from build123d import *

# Parameters (mm, degrees)
BOSS_EXTRUDE1_DEPTH = 0.5
BOSS_EXTRUDE6_DEPTH = 5
BOSS_EXTRUDE5_DEPTH = 6.75
LPATTERN2_COUNT     = 2
LPATTERN2_PITCH     = 13.75
CUT_EXTRUDE4_REACH  = 84.156
SKETCH10_R          = 1.75
LPATTERN3_COUNT     = 2
LPATTERN3_PITCH     = 12
CUT_EXTRUDE5_REACH  = 84.156
SKETCH12_R          = 1.25
SKETCH13_W          = 7
SKETCH13_H          = 6
CUT_EXTRUDE6_DEPTH  = 1
CHAMFER1_SIZE       = 5
CUT_EXTRUDE8_REACH  = 84.105
SKETCH15_W          = 10
SKETCH15_H          = 3
CUT_EXTRUDE9_REACH  = 84.032
SKETCH16_W          = 3
SKETCH16_H          = 7


with BuildPart() as part:
    # Sketch1 → Boss-Extrude1 (new, symmetric)
    with BuildSketch(Plane.XY):
        with BuildLine():
            Line((-56.5, -6), (27.587658385, -6))
            Line((27.587658385, -6), (27.587658385, 0))
            ThreePointArc((27.587658385, 0), (37.034297035, 20.970760182), (59, 27.791292246))
            Line((59, 27.791292246), (76, 25.703954711))
            Line((76, 25.703954711), (76, 30.62))
            Line((76, 30.62), (0, 30.62))
            Line((0, 30.62), (0, -2.5))
            Line((0, -2.5), (-56.5, -2.5))
            Line((-56.5, -2.5), (-56.5, -6))
        make_face()
    extrude(amount=BOSS_EXTRUDE1_DEPTH, both=True)

    # Sketch5 → Boss-Extrude6 (add)
    with BuildSketch(Plane(origin=(0, 0, 0), x_dir=(1, 0, 0), z_dir=(0, 1, 0))):
        with BuildLine():
            Line((0, 0.5), (3, 0.5))
            ThreePointArc((3, 0.5), (0, 3.5), (-3, 0.5))
            Line((-3, 0.5), (-3, -0.5))
            Line((-3, -0.5), (0, -0.5))
            Line((0, -0.5), (0, 0.5))
        make_face()
    boss_extrude6 = extrude(amount=BOSS_EXTRUDE6_DEPTH)

    # Sketch9 → Boss-Extrude5 (add)
    with BuildSketch(Plane.ZY):
        with BuildLine():
            Line((-0.5, 30.62), (-3, 30.62))
            ThreePointArc((-3, 30.62), (-6, 27.62), (-3, 24.62))
            Line((-3, 24.62), (-0.5, 24.62))
            Line((-0.5, 24.62), (-0.5, 30.62))
        make_face()
    boss_extrude5 = extrude(amount=-BOSS_EXTRUDE5_DEPTH)

    # LPattern2: Boss-Extrude5 ×2
    with Locations(*[(i * LPATTERN2_PITCH, 0, 0) for i in range(1, LPATTERN2_COUNT)]):
        add(boss_extrude5)

    # Cut-Extrude4: up to this face of the body (flat: up to its plane)
    cut_extrude4_end = Plane(part.part.faces().sort_by_distance((20.5, 27.62, -2.97425968))[0])
    # Sketch10 → Cut-Extrude4 (cut, up to the picked face)
    with BuildSketch(Plane.ZY, mode=Mode.PRIVATE) as cut_extrude4_sk1:
        with Locations((-3, 27.62)):
            Circle(SKETCH10_R)
    cut_extrude4_tool1 = split(extrude(cut_extrude4_sk1.sketch, amount=-CUT_EXTRUDE4_REACH, mode=Mode.PRIVATE), bisect_by=cut_extrude4_end, keep=Keep.BOTH, mode=Mode.PRIVATE)
    add(cut_extrude4_tool1.solids().sort_by(Axis((0, 27.62, -3), (1, 0, 0)))[0], mode=Mode.SUBTRACT)

    # LPattern3: Boss-Extrude6 ×2
    with Locations(*[(0, i * LPATTERN3_PITCH, 0) for i in range(1, LPATTERN3_COUNT)]):
        add(boss_extrude6)

    # Cut-Extrude5: up to this face of the body (flat: up to its plane)
    cut_extrude5_end = Plane(part.part.faces().sort_by_distance((-0.26258716, 17, -1.462819587))[0])
    # Sketch12 → Cut-Extrude5 (cut, up to the picked face)
    with BuildSketch(Plane.XZ, mode=Mode.PRIVATE) as cut_extrude5_sk1:
        with Locations(Location((0, -1.9, 0), (0, 0, 270))):
            Circle(SKETCH12_R)
    cut_extrude5_tool1 = split(extrude(cut_extrude5_sk1.sketch, amount=-CUT_EXTRUDE5_REACH, mode=Mode.PRIVATE), bisect_by=cut_extrude5_end, keep=Keep.BOTH, mode=Mode.PRIVATE)
    add(cut_extrude5_tool1.solids().sort_by(Axis((0, 0, -1.9), (0, 1, 0)))[0], mode=Mode.SUBTRACT)

    # Sketch13 → Cut-Extrude6 (cut)
    with BuildSketch(Plane(origin=(0, 0, -0.5), x_dir=(-1, 0, 0), z_dir=(0, 0, -1))):
        with Locations((-10.25, 27.62)):
            Rectangle(SKETCH13_W, SKETCH13_H)
    extrude(amount=-CUT_EXTRUDE6_DEPTH, mode=Mode.SUBTRACT)

    # Chamfer1
    # the kernel refuses this chamfer: 5 mm, written as the material it takes off along each edge
    with BuildSketch(Plane(origin=(76, 30.62, 13.35841494), x_dir=(-0.9996219169112968, 0.027495876610586282, 0), z_dir=(0, 0, -1))) as chamfer1_piece_1:
        Polygon((CHAMFER1_SIZE * 0.999621916911, -CHAMFER1_SIZE * 0.0274958766106), (-CHAMFER1_SIZE * 0.0274958766106, -CHAMFER1_SIZE * 0.999621916911), (0, 0), align=None)
    extrude(amount=26.71682988, mode=Mode.SUBTRACT)

    # Sketch15 → Cut-Extrude8 (cut, up to next)
    with BuildSketch(Plane.XY.offset(0.5), mode=Mode.PRIVATE) as cut_extrude8_sk1:
        with Locations((40.65429408, 29.12)):
            Rectangle(SKETCH15_W, SKETCH15_H)
    cut_extrude8_tool1 = extrude(cut_extrude8_sk1.sketch, amount=-CUT_EXTRUDE8_REACH, mode=Mode.PRIVATE) & part.part
    add(cut_extrude8_tool1.solids().sort_by_distance((40.654294, 29.12, 0.5))[0], mode=Mode.SUBTRACT)

    # Sketch16 → Cut-Extrude9 (cut, up to next)
    with BuildSketch(Plane(origin=(0, 0, -0.5), x_dir=(-1, 0, 0), z_dir=(0, 0, -1)), mode=Mode.PRIVATE) as cut_extrude9_sk1:
        with Locations((-1.5, 8.5)):
            Rectangle(SKETCH16_W, SKETCH16_H)
    cut_extrude9_tool1 = extrude(cut_extrude9_sk1.sketch, amount=-CUT_EXTRUDE9_REACH, mode=Mode.PRIVATE) & part.part
    add(cut_extrude9_tool1.solids().sort_by_distance((1.5, 8.5, -0.5))[0], mode=Mode.SUBTRACT)


solid = part.part
Part model, mm, in its own coordinate system. A direction names the side the tool comes from. Coordinates: 2 decimals unless noted, no trailing zeros. Write each loop counter-clockwise with the first axis right and the second up, starting at its lowest first coordinate (ties: lowest second). Pieces come first, ordered by that corner, then holes. Notation, with made-up numbers: (75, 24) - (115, 24) arc R26 ccw to (115, 47) - close; hole circle Ø9 at (78, 81). An arc over 180 degrees is marked (long way). Put each result on its own line as item: value.
1. Band-saw the part on A-A (x = 22.5). Write the cut outline in (y, z).
Final values:
outline: (-6, -0.5) - (30.62, -0.5) - (30.62, 0.5) - (-6, 0.5) - close
2. Band-saw the part on B-B (y = 20.5). Write the cut outline in (x, z).
Final values:
outline: (0, -0.5) - (36.52, -0.5) - (36.52, 0.5) - (0, 0.5) - close
3. Flat gauge pins, fed straight in: pin 1 Ø1.8 at (y, z) = (28, -4) entering from +X; pin 2 Ø0.5 at (x, z) = (12, 0) entering from +Y; pin 3 Ø1.1 at (x, z) = (-23, 0) entering from +Y; pin 4 Ø3 at (y, z) = (27.62, -3) entering from +X. Where does each tip first touch, or does it go through?
Final values:
pin 1: stops at x = 20.5
pin 2: stops at y = 24.62
pin 3: stops at y = -2.5
pin 4: passes through
4. Two-plate mould, pull along Z, no slides. Class faces 1 (the flat face through (-0.7, 0, -0.6)), 2 (the cylindrical face through (-0.479, 14.465, -3.055)), 3 (the cylindrical face through (0.1, 2.5, -3.5)): +Z half, -Z half, draft (parallel to the pull), parting line (faces both ways), or undercut.
Final values:
face 1: draft
face 2: undercut
face 3: -Z half
5. 3-axis set-ups, long thin cutter, end or side, ignore diameter. For faces 4 (the flat face through (0, 27, -1)), 5 (the flat face through (0.7, 12, -0.6)), 6 (the flat face through (67.33, 26.77, 0.01)): which of +Z, -Z, +X, -X, +Y, -Y reach the whole face in a straight line?
Final values:
face 4: +Z, -Z, -X, +Y
face 5: +Z, -Z, -X
face 6: +Z, -Z, -Y
6. Probe line 1 along Y through (x, z) = (19, -2.75); line 2 along X through (y, z) = (25.5, -0.75); line 3 along Y through (x, z) = (17.5, -4.25). List the from-to ranges inside material, lowest first. Write a range as [from, to].
Final values:
line 1: y = [24.62, 25.89], [29.35, 30.62]
line 2: x = [0, 6.75], [13.75, 20.5]
line 3: y = [24.89, 26.4], [28.84, 30.35]
